Autodesk Inventor part; units mm, degrees
ref_plane "YZ Plane" through (0, 0, 0) normal (1, 0, 0) x (0, 1, 0)
ref_plane "XZ Plane" through (0, 0, 0) normal (0, 1, 0) x (-1, 0, 0)
ref_plane "XY Plane" through (0, 0, 0) normal (0, 0, 1) x (1, 0, 0)
sketch "Esboço1" plane through (0, 0, 0) normal (1, 0, 0) x (0, 1, 0)
  circle A0 centre (0, 0) radius 20
  circle A1 centre (0, 0) radius 37.5
  dimension "d0" = 40
  dimension "d1" = 75
extrude "Extrusão1" add sketch "Esboço1" along normal blind 5
sketch "Esboço3" plane through (5, 0, 0) normal (1, 0, 0) x (0, 0, -1)
  line L0 (154.1962, 109.7603) -> (153.014, 111.1125)
  line L1 (40.5387, 95.9825) -> (78.7824, 129.4199)
  line L2 (153.014, 111.1125) -> (-99.3237, 399.7205)
  circle A0 centre (0, 0) radius 37.5
  line L3 (-28.231, -24.6832) -> (-242.5302, 220.4188)
  arc A1 (-100.8216, 158.3529) -> (38.988, 202.8563) centre (-40.5953, 211.0103) ccw
  line L4 (-100.8216, 158.3529) -> (-166.6433, 233.6357)
  line L5 (-166.6433, 233.6357) -> (-204.2865, 253.8562)
  circle A2 centre (46.9464, 202.0409) radius 2.5
  circle A3 centre (36.4428, 168.4765) radius 2.5
  arc A4 (52.969, 207.3066) -> (38.988, 202.8563) centre (46.9464, 202.0409) ccw
  line L6 (52.969, 207.3066) -> (85.8799, 169.6652)
  line L7 (85.8799, 169.6652) -> (14.3612, 107.1346)
  line L8 (14.3612, 107.1346) -> (36.5877, 8.2215)
  circle A5 centre (-224.6099, 219.2172) radius 2.5
  circle A6 centre (-205.4881, 235.936) radius 2.5
  circle A7 centre (-215.049, 227.5766) radius 2.5
  line L9 (-242.5302, 220.4188) -> (-204.2865, 253.8562)
  dimension "d5" = 160
  dimension "d10" = 100
  dimension "d11" = 5
  dimension "d12" = 5
  dimension "d13" = 88
  dimension "d14" = 88
  dimension "d15" = 20
  dimension "d16" = 50
  dimension "d18" = 50
  dimension "d19" = 95
  dimension "d20" = 5
  dimension "d21" = 5
  dimension "d22" = 5
  dimension "d23" = 12.7
  dimension "d25" = 12.7
  dimension "d30" = 280
  dimension "d31" = 140
  dimension "d32" = 12.7
  dimension "d33" = 12.7
  dimension "d34" = 12.7
  dimension "d35" = 12.7
extrude "Extrusão2" add sketch "Esboço3" against normal blind 5 contours A0 L3 L9 L5 L4 A1 A4 L6 L7 L8
sketch "Esboço4" plane through (5, 0, 0) normal (1, 0, 0) x (0, 0, -1)
  line L0 (154.1962, 109.7603) -> (153.014, 111.1125)
  line L1 (153.014, 111.1125) -> (-112.9577, 415.3142)
  circle A0 centre (-34.8401, 212.0241) radius 75
  circle A1 centre (-121.7601, 171.9256) radius 20
  line L2 (-204.2865, 253.8562) -> (-242.5302, 220.4188)
  line L3 (-242.5302, 220.4188) -> (-28.231, -24.6832)
  circle A2 centre (-121.7601, 171.9256) radius 2.5
  circle A3 centre (-173.5863, 191.7005) radius 5
  circle A4 centre (-22.3357, 17.5375) radius 2.5
  circle A5 centre (-27.4315, -7.3461) radius 2.5
  circle A6 centre (22.3357, -17.5375) radius 2.5
  circle A7 centre (27.4315, 7.3461) radius 2.5
  point P0 (0, 0)
  dimension "d38" = 150
  dimension "d39" = 40
  dimension "d40" = 116
  dimension "d41" = 59
  dimension "d42" = 5
  dimension "d43" = 10
  dimension "d45" = 33
  dimension "d46" = 67
extrude "Extrusão3" cut sketch "Esboço4" against normal blind 5 contours A2 | A3 | A4 | A5 | A6 | A7
sketch "Esboço5" plane through (5, 0, 0) normal (1, 0, 0) x (0, 0, -1)
  circle A0 centre (-166.0206, 215.9476) radius 2.5193 construction
  circle A1 centre (-197.8334, 199.2662) radius 2.5193
  circle A2 centre (-149.3392, 184.1348) radius 2.5193
  circle A3 centre (-166.0206, 215.9476) radius 2.5193
  circle A4 centre (-181.152, 167.4534) radius 2.5193
  point P0 (0, 0)
extrude "Extrusão4" cut sketch "Esboço5" against normal blind 10
sketch "Esboço6" plane through (5, 0, 0) normal (1, 0, 0) x (0, 0, -1)
  line L0 (78.9782, 129.7261) -> (84.3768, 134.4529)
  line L1 (85.8799, 169.6652) -> (14.3612, 107.1346)
  line L2 (89.2225, 138.7154) -> (85.8799, 169.6652)
  line L3 (77.937, 128.8343) -> (47.698, 136.2818)
  line L4 (77.937, 128.8343) -> (89.2225, 138.7154)
  point P0 (0, 0)
  dimension "d58" = 55
  dimension "d61" = 15
  dimension "d62" = 25.5
  dimension "d64" = 55
extrude "Extrusão5" add sketch "Esboço6" against normal blind 5
fillet "Arredondamento1" radius 5 8 edges at (2.5, 107.1346, -14.3612) (2.5, 136.2818, -47.698) (2.5, 128.8343, -77.937) (2.5, 138.7154, -89.2225) (2.5, 169.6652, -85.8799) (2.5, 233.6357, 166.6433) (2.5, 253.8562, 204.2865) (2.5, 220.4188, 242.5302)
equation "\"d25\" = d23"
equation "\"d64\" = d58"
properties part number "CHAPA LATERAL INTAKE V2"
Work out the finished part from the listing and answer in its coordinate system (mm). A direction names the side the tool comes from. Give positions to 0.01 mm unless a question says otherwise; leave off trailing zeros. Loops run counter-clockwise (first coordinate to the right, second up) from the corner with the lowest first, then second, coordinate; pieces in that order, holes last. Notation, with made-up numbers: (-36, -13.5) - (-13, -13.5) arc R23 ccw to (-13, 8.5) - close; hole circle Ø3 at (-17, -6). An arc over 180 degrees is marked (long way). Answer in a Markdown table with one row per item.
(1) Section C-C (x = 1.75) is taken. State how many separate pieces and enclosed holes the cut face has, and give its area (3 significant figures).
Results list:
| item | result |
|---|---|
| separate pieces | 1 |
| enclosed holes | 16 |
| area | 32,100 mm² |
(2) For a pull along Z with two mould halves and no side action, classify faces 4 (the face through (2.535, 243.015, 184.103)), 5 (the face through (3, 94, 132)), 6 (the face through (2.535, 134.395, 17.572)), 7 (the face through (2.465, -4.336, 19.524)) as pulls with the +Z half, pulls with the -Z half, needs draft (parallel to the pull), parting line crosses it, or undercut.
Results list:
| item | result |
|---|---|
| face 4 | pulls with the -Z half |
| face 5 | pulls with the +Z half |
| face 6 | undercut |
| face 7 | undercut |
(3) Flat-ended cylindrical pins translate along their axes: pin 1 Ø3 at (y, z) = (215.95, 166.02) entering from +X; pin 2 Ø2 at (x, z) = (1, 65) entering from -Y; pin 3 Ø1 at (x, z) = (1.5, 56.5) entering from +Y; pin 4 Ø2 at (x, y) = (2.5, 205.5) entering from -Z. Find the tip coordinate at first contact, or state that the pin passes through.
Results list:
| item | result |
|---|---|
| pin 1 | passes through |
| pin 2 | stops at y = 16.23 |
| pin 3 | stops at y = 132.71 |
| pin 4 | stops at z = -55.42 |
(4) Section B-B (z = 0) is taken. Give the vertices of the cut face in (x, y).
Results list:
| item | result |
|---|---|
| outline | (0, -37.5) - (5, -37.5) - (5, -20) - (0, -20) - close; (0, 20) - (5, 20) - (5, 142.08) - (0, 142.08) - close |
(5) Section A-A (y = 0) is taken. Give the vertices of the cut face in (x, z), and give its area (3 significant figures).
Results list:
| item | result |
|---|---|
| outline | (0, -37.5) - (5, -37.5) - (5, -20) - (0, -20) - close; (0, 20) - (5, 20) - (5, 49.81) - (0, 49.81) - close |
| area | 237 mm² |
(6) Consider L1, parallel to Z at x = 2.8, y = 201; L2, parallel to Z at x = 4.4, y = 2.5; L3, parallel to Z at x = 3.75, y = 2. Determine where each line is inside the solid, lowest interval first. Write a range as [from, to].
Results list:
| item | result |
|---|---|
| L1 | z = [-58.48, -49.22], [-44.67, -38.78], [138.11, 196.01], [199.66, 225.55] |
| L2 | z = [-37.42, -19.84], [19.84, 52] |
| L3 | z = [-37.45, -19.9], [19.9, 51.56] |
(7) A tool of negligible diameter and unlimited length cuts with its end or side. For faces 1 (the face through (2.535, 195.13, 132.977)), 2 (the face through (2.54, 56.9, -25.65)), 3 (the face through (2.535, 122.009, -31.374)), from which of +Z, -Z, +X, -X, +Y, -Y can it reach the whole face along a straight path? Write none if from no direction.
Results list:
| item | result |
|---|---|
| face 1 | +X, -X, +Y |
| face 2 | -Z, +X, -X |
| face 3 | +X, -X |
(8) Section D-D (z = 34) is taken. Give the vertices of the cut face in (x, y).
Results list:
| item | result |
|---|---|
| outline | (0, -18.08) - (5, -18.08) - (5, 131.28) - (0, 131.28) - close |
